Build history of the part. All positions in model axes, mm. Face numbers are marked on the shaded views. A direction names the side the tool comes from. Round coordinates to 2 decimals unless told otherwise and drop trailing zeros. Loops run counter-clockwise (first coordinate to the right, second up) from the corner with the lowest first, then second, coordinate; pieces in that order, holes last. Notation, with made-up numbers: (66.5, -27) - (118.5, -27) arc R33 cw to (118.5, 3) - close; hole circle Ø11 at (11.25, -6.5). An arc over 180 degrees is marked (long way). Use a Markdown table: item, result.
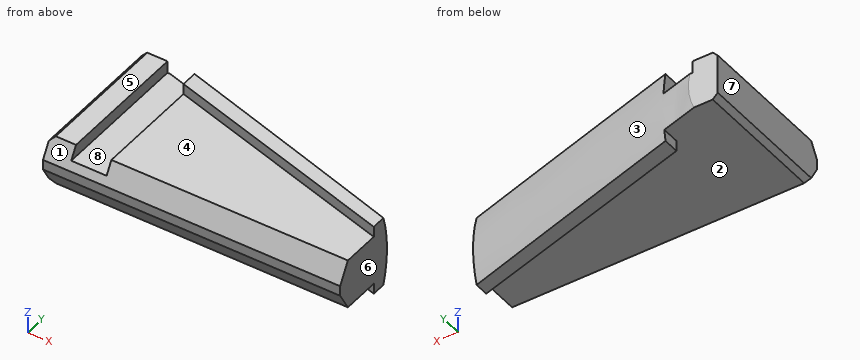
from build123d import *

# Parameters (mm, degrees)
R_VOLUTION1_ANGLE       = 180
ESQUISSE3_OUTSIDE_W     = 53.726
ESQUISSE3_OUTSIDE_H     = 33.296
ENL_V_MAT_EXTRU_1_DEPTH = 42.220813774
ESQUISSE4_W             = 1.05
ESQUISSE4_H             = 30
ESQUISSE6_W             = 6
ESQUISSE6_H             = 1.05
ENL_V_MAT_EXTRU_2_DEPTH = 33.923699671
CHANFREIN1_SIZE         = 0.5


with BuildPart() as part:
    # Esquisse1 → Révolution1 (revolve, symmetric)
    with BuildSketch(Plane.XY) as r_volution1_sk:
        Polygon((0, 20.430314341), (0, 0), (29.4, 0), (29.4, 12), align=None)
    revolve(axis=Axis((0, 0, 0), (-1, 0, 0)), revolution_arc=R_VOLUTION1_ANGLE / 2)
    revolve(r_volution1_sk.sketch, axis=Axis((0, 0, 0), (1, 0, 0)), revolution_arc=R_VOLUTION1_ANGLE / 2)

    # Esquisse3 outside → Enlèv. mat.-Extru.1 (cut, through all)
    with BuildSketch(Plane(origin=(29.4, 0, 0), x_dir=(0, 0, -1), z_dir=(1, 0, 0))):
        with Locations((0, 10.215)):
            Rectangle(ESQUISSE3_OUTSIDE_W, ESQUISSE3_OUTSIDE_H)
        Polygon((-3.5, 6.932050808), (-0.5, 5.2), (0.5, 5.2), (3.5, 6.932050808), (3.5, 19.6), (-3.5, 19.6), align=None, mode=Mode.SUBTRACT)
    extrude(amount=-ENL_V_MAT_EXTRU_1_DEPTH, mode=Mode.SUBTRACT)

    # Enlèvement de matière-Balayage1: sweep along a path in Esquisse5
    with BuildLine(Plane(origin=(0, 0, 0), x_dir=(-1, 0, 0), z_dir=(0, 0, -1))) as enl_vement_de_mati_re_balayage1_path:
        Line((-29.4, 10.078240283), (0, 18.508554625))
    # Esquisse4 → Enlèvement de matière-Balayage1 (sweep, cut)
    with BuildSketch(Plane(origin=(29.4, 0, 0), x_dir=(0, 0, -1), z_dir=(1, 0, 0))):
        with Locations((2.975, -4.921759717)):
            Rectangle(ESQUISSE4_W, ESQUISSE4_H)
        with Locations((-2.975, -4.921759717)):
            Rectangle(ESQUISSE4_W, ESQUISSE4_H)
    sweep(path=enl_vement_de_mati_re_balayage1_path.line, mode=Mode.SUBTRACT)

    # Esquisse6 → Enlèv. mat.-Extru.2 (cut, through all)
    with BuildSketch(Plane(origin=(0, 19.6, 0), x_dir=(-1, 0, 0), z_dir=(0, 1, 0))):
        with Locations((-3, -2.975)):
            Rectangle(ESQUISSE6_W, ESQUISSE6_H)
        Polygon((0, 3.5), (-6, 3.5), (-6, 2.45), (-6, 1.25), (-2.5, 1.25), (-2.5, 2.45), (0, 2.45), align=None)
    extrude(amount=-ENL_V_MAT_EXTRU_2_DEPTH, mode=Mode.SUBTRACT)

    # Chanfrein1
    chanfrein1_edges = [part.edges().sort_by_distance(p)[0] for p in [
        (0, 12.962916512, -2.45),
        (0, 12.962916512, 2.45),
    ]]
    chamfer(chanfrein1_edges, length=CHANFREIN1_SIZE)


solid = part.part
Q1. Cut at A-A, the plane y = 9.75. List the corners of the cut face in (x, z), plus the area to 3 significant figures.
Results found:
| item | result |
|---|---|
| outline | (0, -1.95) - (0.5, -2.45) - (29.4, -2.45) - (29.4, 2.45) - (6, 2.45) - (6, 1.25) - (2.5, 1.25) - (2.5, 2.45) - (0.5, 2.45) - (0, 1.95) - close |
| area | 140 mm2 |
Q2. Which spindle directions (+Z, -Z, +X, -X, +Y, -Y) get a long thin tool onto all of the face, cutting with end or side? Do the marked faces 1, 2, 3, 4 and 5. Say none if no direction does.
Results found:
| item | result |
|---|---|
| face 1 | +Z, +X, -X, -Y |
| face 2 | -Z, -X, -Y |
| face 3 | +X, +Y |
| face 4 | +Z, -X, -Y |
| face 5 | +Z, -X, +Y, -Y |
Q3. Pull direction X, two halves, no side cores. Call the marked faces 6, 7 and 8: pulls with the +X half, pulls with the -X half, needs draft (parallel to the pull), parting line crosses it, or undercut.
Results found:
| item | result |
|---|---|
| face 6 | pulls with the +X half |
| face 7 | pulls with the -X half |
| face 8 | undercut |
Q4. Drop flat-ended pins along their axis: pin 1 (1 mm diameter, centred on x = 1.5, y = 13.5, fed in from +Z); pin 2 (0.8 mm diameter, centred on y = 18, z = -3, fed in from -X); pin 3 (4 mm diameter, centred on x = 14.5, y = 10.5, fed in from -Z). Give the stop position or say it passes through.
Results found:
| item | result |
|---|---|
| pin 1 | stops at z = 2.45 |
| pin 2 | stops at x = 6 |
| pin 3 | stops at z = -2.45 |
Q5. Cut at D-D, the plane x = 4.5. List the corners of the cut face in (y, z).
Results found:
| item | result |
|---|---|
| outline | (5.2, -0.5) - (6.33, -2.45) - (18.98, -2.45) arc R19.14 ccw to (19.1, 1.25) - (5.63, 1.25) - (5.2, 0.5) - close |
Q6. Cut at B-B, the plane z = 0. List the corners of the cut face in (x, y).
Results found:
| item | result |
|---|---|
| outline | (0, 5.2) - (29.4, 5.2) - (29.4, 12) - (2.9, 19.6) - (0, 19.6) - close |
Q7. Probe line 1 (Z direction, x = 2.25, y = 8.25); line 2 (Z direction, x = 2.75, y = 13.75); line 3 (Y direction, x = 14, z = 0.5). List the from-to ranges inside material, lowest first.
Results found:
| item | result |
|---|---|
| line 1 | z = -2.45 to 2.45 |
| line 2 | z = -2.45 to 1.25 |
| line 3 | y = 5.2 to 16.41 |
Q8. Cut at C-C, the plane x = 15.5. List the corners of the cut face in (y, z), plus the area to 3 significant figures.
Results found:
| item | result |
|---|---|
| outline | (5.2, -0.5) - (6.33, -2.45) - (14.06, -2.45) - (14.06, -3.5) - (15.6, -3.5) arc R15.99 ccw to (15.6, 3.5) - (14.06, 3.5) - (14.06, 2.45) - (6.33, 2.45) - (5.2, 0.5) - close |
| area | 53.8 mm2 |
